Part model, mm, in its own coordinate system. A direction names the side the tool comes from. Round coordinates to 2 decimals unless told otherwise and drop trailing zeros. Loops run counter-clockwise (first coordinate to the right, second up) from the corner with the lowest first, then second, coordinate; pieces in that order, holes last.
Autodesk Inventor part; units mm, degrees
ref_plane "YZ Plane" through (0, 0, 0) normal (1, 0, 0) x (0, 1, 0)
ref_plane "XZ Plane" through (0, 0, 0) normal (0, 1, 0) x (-1, 0, 0)
ref_plane "XY Plane" through (0, 0, 0) normal (0, 0, 1) x (1, 0, 0)
sketch "Sketch3" plane through (0, 0, 0) normal (1, 0, 0) x (0, 1, 0)
  line L0 (0, 190.5) -> (127, 50.8)
  line L1 (0, 139.7) -> (127, 0)
  line L2 (127, 50.8) -> (127, 0)
  line L3 (0, 139.7) -> (0, 190.5)
  point P0 (0, 0)
  dimension "d10" = 34.1718
  dimension "d11" = 42.274
  dimension "d12" = 127
extrude "Extrusion1" add sketch "Sketch3" along normal blind 25.4
sketch "Sketch4" plane through (0, 127, 50.8) normal (0, 1, 0) x (1, 0, 0)
  line L0 (0, -139.7) -> (0, 0)
  line L1 (25.4, 0) -> (25.4, -139.7)
  line L2 (0, 50.8) -> (25.4, 50.8)
  line L3 (0, -139.7) -> (25.4, -139.7)
  line L4 (22.225, 3.175) -> (3.175, 3.175)
  line L5 (3.175, 3.175) -> (3.175, 47.625)
  line L6 (3.175, 47.625) -> (22.225, 47.625)
  line L7 (22.225, 47.625) -> (22.225, 3.175)
  line L8 (0, 0) -> (0, 50.8)
  line L9 (0, 0) -> (25.4, 0)
  dimension "d19" = 3.175
  dimension "d20" = 3.175
  dimension "d21" = 3.175
  dimension "d22" = 19.05
sketch "Sketch6" plane through (0, 0, 139.7) normal (0, -1, 0) x (1, 0, 0)
  line L0 (22.225, 47.625) -> (3.175, 47.625)
  line L1 (3.175, 47.625) -> (3.175, 3.175)
  line L2 (3.175, 3.175) -> (22.225, 3.175)
  line L3 (22.225, 3.175) -> (22.225, 47.625)
  line L4 (25.4, 50.8) -> (25.4, 0)
  line L5 (0, 0) -> (25.4, 0)
  line L6 (0, 50.8) -> (25.4, 50.8)
  point P0 (0, -139.7)
  dimension "d27" = 19.05
  dimension "d28" = 3.175
  dimension "d29" = 3.175
  dimension "d30" = 3.175
sketch3d "3D Sketch1"
  line L0 (25.4, 0, 190.5) -> (25.4, 127, 50.8)
sweep "Sweep1" cut profiles "Sketch6" path "3D Sketch1"
equation "\"d28\" = d19"
equation "\"d29\" = d20"
equation "\"d30\" = d20"
properties part number "Diagonal Roller Cage Support"
1) Slice it at D-D, the plane z = 93. Give the cut face in (x, y) (3 decimals), then the cut area to 3 significant figures.
Values:
outline: (0, 42.455) - (25.4, 42.455) - (25.4, 88.636) - (0, 88.636) - close; hole (3.175, 45.341) - (22.225, 45.341) - (22.225, 85.75) - (3.175, 85.75) - close
area: 403 mm2
2) Slice it at B-B, the plane z = 15.5. Give the cut face in (x, y) (3 decimals).
Values:
outline: (0, 112.909) - (25.4, 112.909) - (25.4, 127) - (22.225, 127) - (22.225, 115.795) - (3.175, 115.795) - (3.175, 127) - (0, 127) - close
3) Tool access for faces 4 (the face through (0, 58, 96)), 5 (the face through (12.833, 64.389, 116.497)): list every direction of +Z, -Z, +X, -X, +Y, -Y with a clear straight run to the whole face (end or side of a thin tool).
Values:
face 4: +Z, -Z, -X, +Y, -Y
face 5: none
4) Drop flat-ended pins along their axis: pin 1 Ø2 at (x, y) = (14.5, 111) entering from +Z; pin 2 Ø2 at (x, y) = (13, 60) entering from -Z; pin 3 Ø6 at (x, z) = (17.5, 111.5) entering from -Y. Give the stop position or say it passes through.
Values:
pin 1: stops at z = 69.5
pin 2: stops at z = 72.6
pin 3: stops at y = 22.91
5) Slice it at A-A, the plane x = 18.5. Give the cut face in (y, z) (3 decimals).
Values:
outline: (0, 139.7) - (127, 0) - (127, 3.175) - (0, 142.875) - close; (0, 187.325) - (127, 47.625) - (127, 50.8) - (0, 190.5) - close
6) Slice it at C-C, the plane y = 25. Give the cut face in (x, z) (3 decimals), then the cut area to 3 significant figures.
Values:
outline: (0, 112.2) - (25.4, 112.2) - (25.4, 163) - (0, 163) - close; hole (3.175, 115.375) - (22.225, 115.375) - (22.225, 159.825) - (3.175, 159.825) - close
area: 444 mm2
7) Wall check: line 1 along X through (y, z) = (117, 43) (3 decimals); line 2 along Y through (x, z) = (21.75, 94.5); line 3 along Z through (x, y) = (16.5, 53) (3 decimals). Give the ranges that are in metal, low to high.
Values:
line 1: x = 0 to 3.175, 22.225 to 25.4
line 2: y = 41.09 to 43.98, 84.39 to 87.27
line 3: z = 81.4 to 84.575, 129.025 to 132.2
8) Mould opens along Z. For faces 1 (the face through (12.52, 62.61, 121.63)), 2 (the face through (12.52, 62.61, 70.83)), 3 (the face through (3.175, 64, 96)) say: released by +Z, released by -Z, zero draft, split by the parting line, or undercut.
Values:
face 1: released by +Z
face 2: released by -Z
face 3: undercut
